Here's how the part is built. I have some questions about the finished solid (model axes, mm). A direction names the side the tool comes from. Coordinates: 2 decimals unless noted, no trailing zeros. Loops run counter-clockwise (first coordinate to the right, second up) from the corner with the lowest first, then second, coordinate; pieces in that order, holes last. Notation, with made-up numbers: (-34.5, 48.5) -> (20.5, 48.5) arc R14 ccw to (20.5, 66.5) -> close; hole circle Ø3 at (-27, 33.25). An arc over 180 degrees is marked (long way). Answer as a JSON object with one key per item and string values. Group by question number.
1) I want a section at D-D (x = 2.25). Write out the boundary of the cut face in (y, z), then the cut area to 3 significant figures.
2) I'm going to push flat-ended pins straight in: pin 1 (5 mm diameter, centred on x = 5.5, y = 4.5, fed in from -Z); pin 2 (2 mm diameter, centred on x = 7.5, y = 0.5, fed in from -Z); pin 3 (1.5 mm diameter, centred on x = 2, z = -3, fed in from -Y). Where does each tip first touch, or does it pass through?
3) I want a section at C-C (z = 5.25). Write out the boundary of the cut face in (x, y) (3 decimals).
4) Which directions (+Z, -Z, +X, -X, +Y, -Y) give clear straight access to the entire face, cutting with the end or side of a thin tool? Please do faces 1 (the cylindrical face through (1.976, 0.045, 4.42)), 2 (the cylindrical face through (9.38, -0.01, -4.05)), 3 (the cylindrical face through (9.38, 4.05, -0.01)).
5) I need wall thicknesses on probe 1 along X at (y, z) = (4.1, 0) (3 decimals); probe 2 along Y at (x, z) = (8.75, 0); probe 3 along Y at (x, z) = (1.5, 0). Which ranges of each line are inside material? Lowest first, please. Write a range as [from, to].
6) If we mould it in two halves opening along X, with no side actions, what happens to faces 4 (the cylindrical face through (9.377, -1.558, -3.738)), 5 (the flat face through (0, 0, -3)), 6 (the flat face through (14, 0, -3))? For each: +X half, -X half, draft (parallel to the pull), parting line (faces both ways), or undercut.
7) I want a section at A-A (z = 0). Write out the boundary of the cut face in (x, y) (3 decimals), then the cut area to 3 significant figures.
```python
from build123d import *

# Parameters (mm, degrees)
CROQUIS1_R                               = 6.5
CORPO_LADO_MOTOR_13X6_DEPTH              = 6
CROQUIS3_R                               = 4.8
CORPO_DOS_DENTES_9_6X6_85_DEPTH          = 6.85
CORTE_DO_DENTE_R0_5_REACH                = 13.464
ARREDONDAMENTO_RAIO_0_15MM_R             = 0.15
CORTE_DOS_16_DENTES_COUNT                = 16
ARREDONDAMENTO_RAIO_0_15MM_OF_CORTE_DO_R = 0.15
CROQUIS4_R                               = 6.5
FACE_DIREITA_20_DEPTH                    = 1.15
CROQUIS6_R                               = 2.5
FURO_PASSANTE_5_DEPTH                    = 14
FURO_DE_FIXA_O_1_M2_5_REACH              = 22.18
FURO_DE_FIXA_O_1_M2_5_BORE_R             = 1.025
FURO_DE_FIXA_O_2_M2_5_COUNT              = 2
FURO_DE_FIXA_O_2_M2_5_ANGLE              = 90


with BuildPart() as part:
    # Croquis1 → Corpo Lado Motor - Ø13x6 (new body)
    with BuildSketch(Plane(origin=(0, 0, 0), x_dir=(0, 0, -1), z_dir=(1, 0, 0))):
        Circle(CROQUIS1_R)
    extrude(amount=CORPO_LADO_MOTOR_13X6_DEPTH)

    # Croquis3 → Corpo dos Dentes Ø9.6x6.85 (add)
    with BuildSketch(Plane(origin=(6, 0, 0), x_dir=(0, 0, -1), z_dir=(1, 0, 0))):
        with Locations(Location((0, 0, 0), (0, 0, 180))):
            Circle(CROQUIS3_R)
    extrude(amount=CORPO_DOS_DENTES_9_6X6_85_DEPTH)

    # Croquis5 → Corte do Dente - R0.5 (cut, up to next)
    with BuildSketch(Plane(origin=(6, 0, 0), x_dir=(0, 0, -1), z_dir=(1, 0, 0)), mode=Mode.PRIVATE) as corte_do_dente_r0_5_sk1:
        with BuildLine():
            Line((-0.473505997, 4.389400899), (-0.6, 4.76235236))
            ThreePointArc((-0.6, 4.76235236), (0, 4.8), (0.6, 4.76235236))
            Line((0.6, 4.76235236), (0.473505997, 4.389400899))
            ThreePointArc((0.473505997, 4.389400899), (0, 4.05), (-0.473505997, 4.389400899))
        make_face()
    corte_do_dente_r0_5_tool1 = extrude(corte_do_dente_r0_5_sk1.sketch, amount=CORTE_DO_DENTE_R0_5_REACH, mode=Mode.PRIVATE) & part.part
    corte_do_dente_r0_5 = corte_do_dente_r0_5_tool1.solids().sort_by_distance((6, 4.473914, 0))[0]
    add(corte_do_dente_r0_5, mode=Mode.SUBTRACT)

    # Arredondamento - Raio 0.15mm
    arredondamento_raio_0_15mm_edges = [part.edges().sort_by_distance(p)[0] for p in [
        (9.425, 4.76235236, 0.6),
        (9.425, 4.76235236, -0.6),
    ]]
    fillet(arredondamento_raio_0_15mm_edges, radius=ARREDONDAMENTO_RAIO_0_15MM_R)

    # Corte dos 16 Dentes: Corte do Dente - R0.5 ×16 about axis
    corte_dos_16_dentes_axis = Axis((0, 0, 0), (1, 0, 0))
    for i in range(1, CORTE_DOS_16_DENTES_COUNT):
        add(corte_do_dente_r0_5.rotate(corte_dos_16_dentes_axis, i * 360 / CORTE_DOS_16_DENTES_COUNT), mode=Mode.SUBTRACT)

    # Arredondamento - Raio 0.15mm of Corte do
    arredondamento_raio_0_15mm_of_corte_do_edges = [part.edges().sort_by_distance(p)[0] for p in [
        (9.425, 4.170229813, 2.376801067),
        (9.425, 4.629449931, 1.268145628),
        (9.425, 2.943227579, 3.791755717),
        (9.425, 3.791755717, 2.943227579),
        (9.425, 1.268145628, 4.629449931),
        (9.425, 2.376801067, 4.170229813),
        (9.425, -0.6, 4.76235236),
        (9.425, 0.6, 4.76235236),
        (9.425, -2.376801067, 4.170229813),
        (9.425, -1.268145628, 4.629449931),
        (9.425, -3.791755717, 2.943227579),
        (9.425, -2.943227579, 3.791755717),
        (9.425, -4.629449931, 1.268145628),
        (9.425, -4.170229813, 2.376801067),
        (9.425, -4.76235236, -0.6),
        (9.425, -4.76235236, 0.6),
        (9.425, -4.170229813, -2.376801067),
        (9.425, -4.629449931, -1.268145628),
        (9.425, -2.943227579, -3.791755717),
        (9.425, -3.791755717, -2.943227579),
        (9.425, -1.268145628, -4.629449931),
        (9.425, -2.376801067, -4.170229813),
        (9.425, 0.6, -4.76235236),
        (9.425, -0.6, -4.76235236),
        (9.425, 2.376801067, -4.170229813),
        (9.425, 1.268145628, -4.629449931),
        (9.425, 3.791755717, -2.943227579),
        (9.425, 2.943227579, -3.791755717),
        (9.425, 4.629449931, -1.268145628),
        (9.425, 4.170229813, -2.376801067),
    ]]
    fillet(arredondamento_raio_0_15mm_of_corte_do_edges, radius=ARREDONDAMENTO_RAIO_0_15MM_OF_CORTE_DO_R)

    # Croquis4 → Face Direita Ø20 (add)
    with BuildSketch(Plane(origin=(12.85, 0, 0), x_dir=(0, 0, -1), z_dir=(1, 0, 0))):
        Circle(CROQUIS4_R)
    extrude(amount=FACE_DIREITA_20_DEPTH)

    # Croquis6 → Furo Passante Ø5 (cut)
    with BuildSketch(Plane.ZY):
        Circle(CROQUIS6_R)
    extrude(amount=-FURO_PASSANTE_5_DEPTH, mode=Mode.SUBTRACT)

    # Furo de Fixação 1 - M2.5 bore → Furo de Fixação 1 - M2.5 (cut, up to next)
    with BuildSketch(Plane(origin=(0, 6.5, 0), x_dir=(1, 0, 0), z_dir=(0, 1, 0)), mode=Mode.PRIVATE) as furo_de_fixa_o_1_m2_5_sk1:
        with Locations((3, 0)):
            Circle(FURO_DE_FIXA_O_1_M2_5_BORE_R)
    furo_de_fixa_o_1_m2_5_tool1 = extrude(furo_de_fixa_o_1_m2_5_sk1.sketch, amount=-FURO_DE_FIXA_O_1_M2_5_REACH, mode=Mode.PRIVATE) & part.part
    furo_de_fixa_o_1_m2_5 = furo_de_fixa_o_1_m2_5_tool1.solids().sort_by_distance((3, 6.5, 0))[0]
    add(furo_de_fixa_o_1_m2_5, mode=Mode.SUBTRACT)

    # Furo de Fixação 2 - M2.5: Furo de Fixação 1 - M2.5 ×2 about axis
    furo_de_fixa_o_2_m2_5_axis = Axis((21.071067812, 0, 0), (1, 0, 0))
    for i in range(1, FURO_DE_FIXA_O_2_M2_5_COUNT):
        add(furo_de_fixa_o_1_m2_5.rotate(furo_de_fixa_o_2_m2_5_axis, i * FURO_DE_FIXA_O_2_M2_5_ANGLE / (FURO_DE_FIXA_O_2_M2_5_COUNT - 1)), mode=Mode.SUBTRACT)


solid = part.part
```
Determined:
{
 "1": {"outline": "(-0.7, 2.4) -> (-0.7, 6.46) arc R6.5 ccw (long way) to (6.46, -0.7) -> (2.4, -0.7) arc R2.5 cw (long way) to start; (0.7, 2.4) arc R2.5 cw to (2.4, 0.7) -> (6.46, 0.7) arc R6.5 ccw to (0.7, 6.46) -> close", "area": "102 mm^2"},
 "2": {"pin 1": "z = -6.18", "pin 2": "z = -4.75", "pin 3": "y = -6.1"},
 "3": {"outline": "(0, -3.832) -> (6, -3.832) -> (6, 3.832) -> (0, 3.832) -> close; (12.85, -3.832) -> (14, -3.832) -> (14, 3.832) -> (12.85, 3.832) -> close; hole circle Ø2.05 at (3, 0)"},
 "4": {"face 1": "+Z", "face 2": "-Z", "face 3": "+Y"},
 "5": {"probe 1": "[0, 1.975], [4.025, 6], [12.85, 14]", "probe 2": "[-4.05, -2.5], [2.5, 4.05]", "probe 3": "[-6.5, -2.5], [2.5, 6.5]"},
 "6": {"face 4": "undercut", "face 5": "-X half", "face 6": "+X half"},
 "7": {"outline": "(0, -6.5) -> (6, -6.5) -> (6, -4.05) -> (12.85, -4.05) -> (12.85, -6.5) -> (14, -6.5) -> (14, -2.5) -> (0, -2.5) -> close; (0, 2.5) -> (1.975, 2.5) -> (1.975, 6.5) -> (0, 6.5) -> close; (4.025, 2.5) -> (14, 2.5) -> (14, 6.5) -> (12.85, 6.5) -> (12.85, 4.05) -> (6, 4.05) -> (6, 6.5) -> (4.025, 6.5) -> close", "area": "70.2 mm^2"}
}
